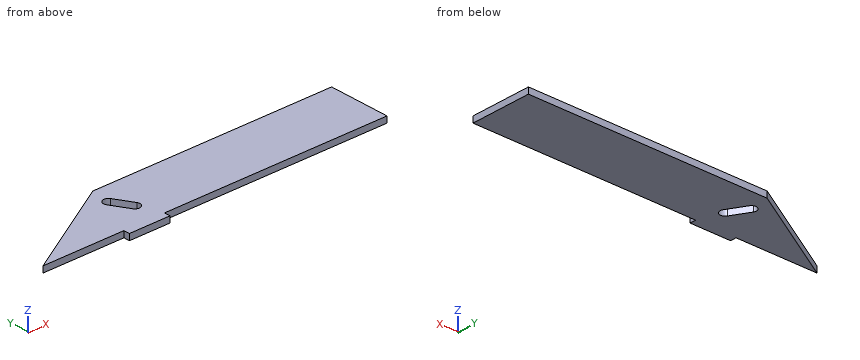
```python
from build123d import *

# Parameters (mm, degrees)
BOSS_EXTRUDE1_DEPTH     = 3
CUT_EXTRUDE3_DEPTH      = 1
CUT_EXTRUDE3_DEPTH_BACK = 3
CUT_EXTRUDE4_DEPTH      = 4
SKETCH6_W               = 3
SKETCH6_H               = 30
BOSS_EXTRUDE2_DEPTH     = 70


with BuildPart() as part:
    # Sketch1 → Boss-Extrude1 (new body)
    with BuildSketch(Plane.XY):
        Polygon((-10, -15), (-10, -18), (10, -18), (10, -15), (50, -15), (50, 15), (-50, 15), (-50, -15), align=None)
    extrude(amount=BOSS_EXTRUDE1_DEPTH)

    # Sketch4 → Cut-Extrude3 (cut, two sides)
    with BuildSketch(Plane.XY.offset(3)) as cut_extrude3_sk:
        Polygon((-50, -14.220304878), (-50, -15), (1.961524227, 15), (-50, 15), align=None)
    extrude(amount=CUT_EXTRUDE3_DEPTH, mode=Mode.SUBTRACT)
    extrude(cut_extrude3_sk.sketch, amount=-CUT_EXTRUDE3_DEPTH_BACK, mode=Mode.SUBTRACT)

    # Sketch5 → Cut-Extrude4 (cut)
    with BuildSketch(Plane.XY.offset(3)):
        with BuildLine():
            Line((7.930435314, -2.338457268), (2.930435314, 6.32179677))
            ThreePointArc((2.930435314, 6.32179677), (-0.484628196, 7.236860279), (-1.399691705, 3.82179677))
            Line((-1.399691705, 3.82179677), (3.600308295, -4.838457268))
            ThreePointArc((3.600308295, -4.838457268), (7.015371804, -5.753520778), (7.930435314, -2.338457268))
        make_face()
    extrude(amount=-CUT_EXTRUDE4_DEPTH, mode=Mode.SUBTRACT)

    # Sketch6 → Boss-Extrude2 (add)
    with BuildSketch(Plane(origin=(50, 0, 0), x_dir=(0, 0, -1), z_dir=(1, 0, 0))):
        with Locations((-1.5, 0)):
            Rectangle(SKETCH6_W, SKETCH6_H)
    extrude(amount=BOSS_EXTRUDE2_DEPTH)


solid = part.part
```
The model under review builds one solid part; all positions refer to its coordinate system, in mm. Round coordinates to 2 decimals unless told otherwise and drop trailing zeros. Loops run counter-clockwise (first coordinate to the right, second up) from the corner with the lowest first, then second, coordinate; pieces in that order, holes last. Notation, with made-up numbers: M 54.25,23.25 L 67.25,23.25 A22 cw 67.25,57.25 Z; hole C 62,61.5 d3. An arc over 180 degrees is marked long. Write item = value, one per line.
Item 1: Take a section at A-A on y = 1.5. Write out the cut boundary in (x, z).
Return value:
outline = M -21.42,0 L -0.06,0 L -0.06,3 L -21.42,3 Z; M 5.71,0 L 120,0 L 120,3 L 5.71,3 Z
Item 2: Take a section at D-D on y = 12. Write out the cut boundary in (x, z), then the cut area to 3 significant figures.
Return value:
outline = M -3.23,0 L 120,0 L 120,3 L -3.23,3 Z
area = 370 mm2
Item 3: Take a section at C-C on x = 31. Write out the cut boundary in (y, z).
Return value:
outline = M -15,0 L 15,0 L 15,3 L -15,3 Z
Item 4: Insertion check: P1, Ø0.9, axis at x = -34.5, z = 1.5, coming from the -Y side. The pin has a flat end and moves straight along its axis. Give the tip position at first contact, or say it passes through.
Return value:
P1 = -15
Item 5: Take a section at B-B on z = 1.5. Write out the cut boundary in (x, y), then the cut area to 3 significant figures.
Return value:
outline = M -50,-15 L -10,-15 L -10,-18 L 10,-18 L 10,-15 L 120,-15 L 120,15 L 1.96,15 Z; hole M -1.4,3.82 L 3.6,-4.84 A2.5 ccw 7.93,-2.34 L 2.93,6.32 A2.5 ccw Z
area = 4,310 mm2
Item 6: For line 1 (Y direction, x = 88.5, z = 2.8); line 2 (X direction, y = 4.5, z = 2.3) (3 decimals); line 3 (X direction, y = -5, z = 1.65), list the stretches that pass through material, from the lowest coordinate up. Write a range as [from, to].
Return value:
line_1 = [-15, 15]
line_2 = [-16.225, -1.668], [3.982, 120]
line_3 = [-32.68, 3.7], [7.83, 120]
